Here's the drawing with two shaded views (mm, measured from the low corner). I have some questions. A direction names the side the tool comes from. Round coordinates to 2 decimals unless told otherwise and drop trailing zeros. Write each loop counter-clockwise with the first axis right and the second up, starting at its lowest first coordinate (ties: lowest second). Pieces come first, ordered by that corner, then holes. Notation, with made-up numbers: (11.5, 65.25) - (16.5, 65.25) arc R25 ccw to (16.5, 90.25) - close; hole circle Ø3 at (33.25, 87.5). An arc over 180 degrees is marked (long way). Return JSON: item names as keys, results as strings. Group by question number.
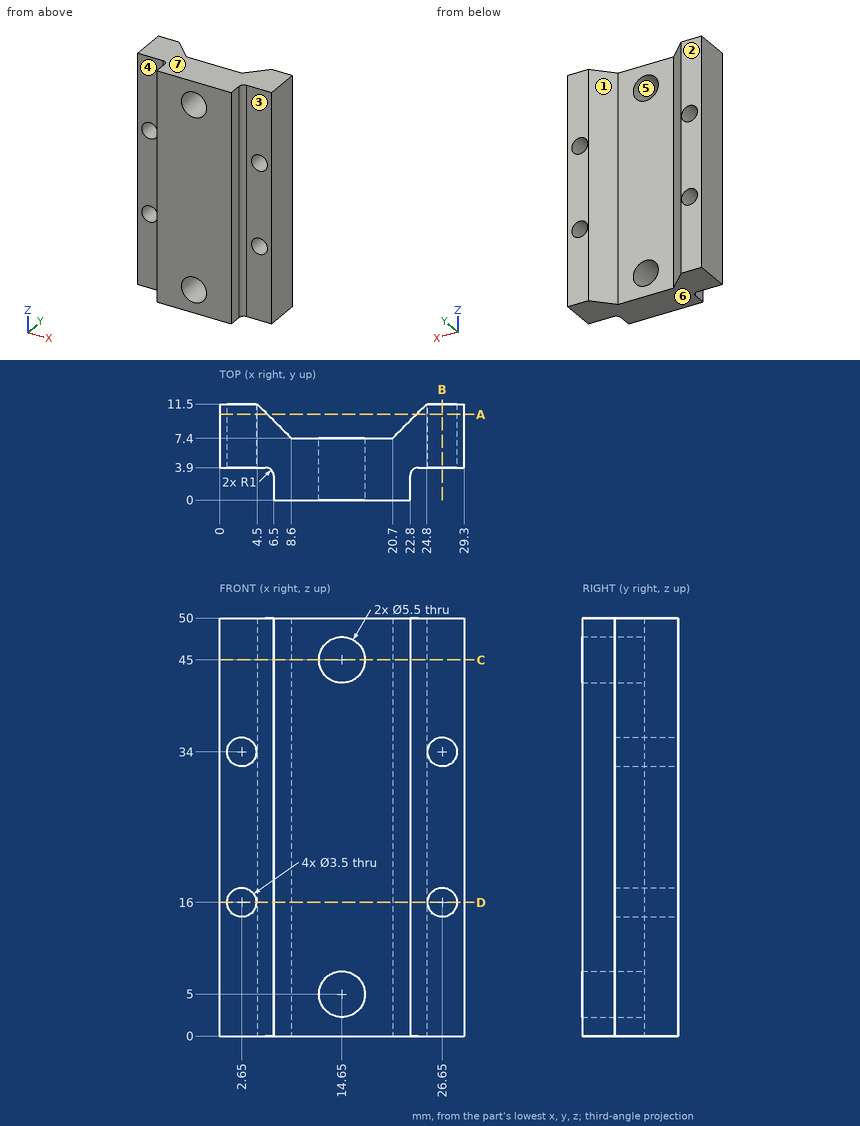
1) Imagine slicing it at A-A (y = 10.25). Please give me the cut outline in (x, z), plus the area to 3 significant figures.
2) If we mould it in two halves opening along Z, with no side actions, what happens to the marked faces 4, 5, 6 and 7? For each: released by +Z, released by -Z, zero draft, split by the parting line, or undercut.
3) For the marked faces 1, 2 and 3, which set-ups out of +Z, -Z, +X, -X, +Y, -Y let a thin tool reach every point of the face, with its end or its side?
4) Will these pins go through, and if not, where does the flat tip stop? pin 1 Ø4.5 at (x, z) = (3, 24) entering from -Y; pin 2 Ø9.5 at (x, z) = (17, 25) entering from +Y; pin 3 Ø4.5 at (x, z) = (14.65, 45) entering from -Y; pin 4 Ø0.9 at (y, z) = (2, 18) entering from +X.
5) Imagine slicing it at C-C (z = 45). Please give me the cut outline in (x, y), plus the area to 3 significant figures.
6) Imagine slicing it at B-B (x = 26.65). Please give me the cut outline in (y, z), plus the area to 3 significant figures.
7) I need wall thicknesses on line 1 along Z through (x, y) = (2.65, 7); line 2 along X through (y, z) = (6, 34); line 3 along X through (y, z) = (2.75, 45). Which ranges of each line are inside material? Lowest first, please.
8) Imagine slicing it at D-D (z = 16). Please give me the cut outline in (x, y).
Results found:
{
 "1": {"outline": "(0, 0) - (5.75, 0) - (5.75, 50) - (0, 50) - close; (23.55, 0) - (29.3, 0) - (29.3, 50) - (23.55, 50) - close; hole circle Ø3.5 at (2.65, 16); hole circle Ø3.5 at (2.65, 34); hole circle Ø3.5 at (26.65, 16); hole circle Ø3.5 at (26.65, 34)", "area": "537 mm²"},
 "2": {"face 4": "zero draft", "face 5": "undercut", "face 6": "released by -Z", "face 7": "released by +Z"},
 "3": {"face 1": "+Z, -Z, +Y", "face 2": "+Z, -Z, +X, -X, +Y", "face 3": "+Z, -Z, +X, -Y"},
 "4": {"pin 1": "stops at y = 3.9", "pin 2": "stops at y = 8.45", "pin 3": "passes through", "pin 4": "stops at x = 22.8"},
 "5": {"outline": "(0, 3.9) - (5.5, 3.9) arc R1 cw to (6.5, 2.9) - (6.5, 0) - (11.9, 0) - (11.9, 7.4) - (8.6, 7.4) - (4.5, 11.5) - (0, 11.5) - close; (17.4, 0) - (22.8, 0) - (22.8, 2.9) arc R1 cw to (23.8, 3.9) - (29.3, 3.9) - (29.3, 11.5) - (24.8, 11.5) - (20.7, 7.4) - (17.4, 7.4) - close", "area": "180 mm²"},
 "6": {"outline": "(3.9, 0) - (11.5, 0) - (11.5, 14.25) - (3.9, 14.25) - close; (3.9, 17.75) - (11.5, 17.75) - (11.5, 32.25) - (3.9, 32.25) - close; (3.9, 35.75) - (11.5, 35.75) - (11.5, 50) - (3.9, 50) - close", "area": "327 mm²"},
 "7": {"line 1": "z = 0 to 14.25, 17.75 to 32.25, 35.75 to 50", "line 2": "x = 0 to 0.9, 4.4 to 24.9, 28.4 to 29.3", "line 3": "x = 6.5 to 11.9, 17.4 to 22.8"},
 "8": {"outline": "(0, 3.9) - (0.9, 3.9) - (0.9, 11.5) - (0, 11.5) - close; (4.4, 3.9) - (5.5, 3.9) arc R1 cw to (6.5, 2.9) - (6.5, 0) - (22.8, 0) - (22.8, 2.9) arc R1 cw to (23.8, 3.9) - (24.9, 3.9) - (24.9, 11.5) - (24.8, 11.5) - (20.7, 7.4) - (8.6, 7.4) - (4.5, 11.5) - (4.4, 11.5) - close; (28.4, 3.9) - (29.3, 3.9) - (29.3, 11.5) - (28.4, 11.5) - close"}
}
